Answer from the drawing. Dimensions are ordinates in mm from the lowest x, y and z of the part. A direction names the side the tool comes from. Give positions to 0.01 mm unless a question says otherwise; leave off trailing zeros. Write each loop counter-clockwise with the first axis right and the second up, starting at its lowest first coordinate (ties: lowest second). Pieces come first, ordered by that corner, then holes. Notation, with made-up numbers: (-26, 59) -> (16, 59) arc R9 cw to (16, 73) -> close; hole circle Ø6 at (-28.75, 41). An arc over 180 degrees is marked (long way). Put each result on its own line as item: value. Start each with the question number.
1) A cutting plane is placed at D-D (x = 4). Write down the section's boundary in (y, z) (1 decimal).
2) A cutting plane is placed at A-A (x = 19.05). Write down the section's boundary in (y, z) (1 decimal).
3) Find the intervals of material crossed by line 1 along Y through (x, z) = (19.05, 2.25) (1 decimal); line 2 along Y through (x, z) = (8.5, 12) (1 decimal); line 3 along Z through (x, y) = (16.5, 27.5), in increasing order. Write a range as from..to.
4) A cutting plane is placed at B-B (y = 6). Write down the section's boundary in (x, z), then the cut area to 3 significant figures.
5) For a pull along Y with two mould halves and no side action, classify the marked faces 1, 2 and 3 as released by +Y, released by -Y, zero draft, split by the parting line, or undercut.
6) Flat-ended cylindrical pins translate along their axes: pin 1 Ø3 at (y, z) = (16, 6) entering from -X (1 decimal); pin 2 Ø6 at (x, y) = (10, 37.5) entering from -Z; pin 3 Ø7 at (y, z) = (17, 6.5) entering from +X; pin 4 Ø15 at (x, y) = (19.05, 9.525) entering from -Z. Find the tip coordinate at first contact, or state that the pin passes through.
7) For the marked faces 4, 5, 6, 7 and 8, determine the directions among +Z, -Z, +X, -X, +Y, -Y from which every point of the face is accessible in a straight line to the end or side of a thin tool.
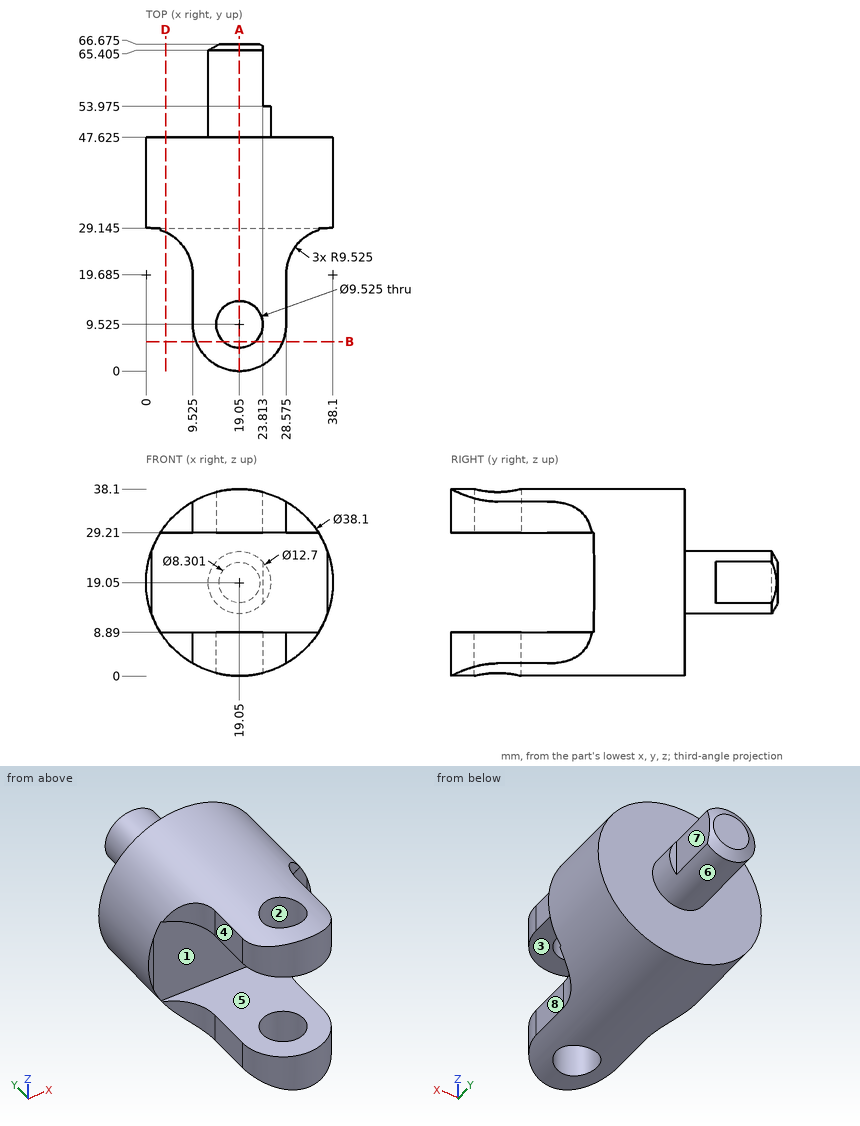
Reply:
1. outline: (28.3, 7.4) -> (47.6, 7.4) -> (47.6, 30.7) -> (28.3, 30.7) -> (28.3, 29.2) -> (29.1, 29.2) -> (29.1, 8.9) -> (28.3, 8.9) -> close
2. outline: (0, 0) -> (4.8, 0) -> (4.8, 8.9) -> (0, 8.9) -> close; (0, 29.2) -> (4.8, 29.2) -> (4.8, 38.1) -> (0, 38.1) -> close; (14.3, 0) -> (47.6, 0) -> (47.6, 12.7) -> (65.4, 12.7) -> (66.7, 14.9) -> (66.7, 23.2) -> (65.4, 25.4) -> (47.6, 25.4) -> (47.6, 38.1) -> (14.3, 38.1) -> (14.3, 29.2) -> (29.1, 29.2) -> (29.1, 8.9) -> (14.3, 8.9) -> close
3. line 1: y = 0..4.8, 14.3..47.6
3. line 2: y = 29.1..47.6
3. line 3: z = 0.17..8.89, 29.21..37.93
4. outline: (10.2, 2.18) arc R19.05 ccw to (15.85, 0.27) -> (15.85, 8.89) -> (10.2, 8.89) -> close; (10.2, 29.21) -> (15.85, 29.21) -> (15.85, 37.83) arc R19.05 ccw to (10.2, 35.92) -> close; (22.25, 0.27) arc R19.05 ccw to (27.9, 2.18) -> (27.9, 8.89) -> (22.25, 8.89) -> close; (22.25, 29.21) -> (27.9, 29.21) -> (27.9, 35.92) arc R19.05 ccw to (22.25, 37.83) -> close
4. area: 177 mm2
5. face 1: released by -Y
5. face 2: undercut
5. face 3: zero draft
6. pin 1: stops at x = 9.5
6. pin 2: stops at z = 0.99
6. pin 3: stops at x = 28.61
6. pin 4: stops at z = 0
7. face 4: +Z, -Z, -X, -Y
7. face 5: +X, -X, -Y
7. face 6: +Y
7. face 7: +Z, -Z, +X, +Y
7. face 8: +Z, -Z, +X, -Y
